Read the model definition and answer for the solid it produces. Units are mm, in the model's axes. Coordinates: 2 decimals unless noted, no trailing zeros. Write each loop counter-clockwise with the first axis right and the second up, starting at its lowest first coordinate (ties: lowest second). Pieces come first, ordered by that corner, then holes. Notation, with made-up numbers: (49, 5.25) -> (84, 5.25) arc R24 cw to (84, 16.25) -> close; hole circle Ø3 at (11, 31.25). An arc over 180 degrees is marked (long way). Return JSON: item names as keys, results as strings.
from build123d import *

# Parameters (mm, degrees)
SKETCH1_R           = 150
BOSS_EXTRUDE1_DEPTH = 10
SKETCH2_R           = 1.73
SKETCH2_R_2         = 2
CUT_EXTRUDE1_DEPTH  = 10


with BuildPart() as part:
    # Sketch1 → Boss-Extrude1 (new body)
    with BuildSketch(Plane(origin=(0, 0, 0), x_dir=(1, 0, 0), z_dir=(0, 1, 0))):
        with Locations(Location((0, 0, 0), (0, 0, 270))):
            Circle(SKETCH1_R)
    extrude(amount=BOSS_EXTRUDE1_DEPTH)

    # Sketch2 → Cut-Extrude1 (cut)
    with BuildSketch(Plane(origin=(0, 10, 0), x_dir=(1, 0, 0), z_dir=(0, 1, 0))):
        with Locations(Location((-14.945, 143.452697854, 0), (0, 0, 270))):
            Circle(SKETCH2_R)
        with Locations(Location((-14.945, 119.392697854, 0), (0, 0, 270))):
            Circle(SKETCH2_R)
        with Locations(Location((14.945, 143.452697854, 0), (0, 0, 90))):
            Circle(SKETCH2_R)
        with Locations(Location((14.945, 119.392697854, 0), (0, 0, 90))):
            Circle(SKETCH2_R)
        with Locations(Location((95.924609368, -72.639098587, 0), (0, 0, 90))):
            Circle(SKETCH2_R)
        with Locations(Location((116.761180583, -84.669098587, 0), (0, 0, 90))):
            Circle(SKETCH2_R)
        with Locations(Location((131.706180583, -58.783599268, 0), (0, 0, 270))):
            Circle(SKETCH2_R)
        with Locations(Location((110.869609368, -46.753599268, 0), (0, 0, 270))):
            Circle(SKETCH2_R)
        with Locations(Location((-110.869609368, -46.753599268, 0), (0, 0, 90))):
            Circle(SKETCH2_R)
        with Locations(Location((-131.706180583, -58.783599268, 0), (0, 0, 90))):
            Circle(SKETCH2_R)
        with Locations(Location((-116.761180583, -84.669098587, 0), (0, 0, 270))):
            Circle(SKETCH2_R)
        with Locations(Location((-95.924609368, -72.639098587, 0), (0, 0, 270))):
            Circle(SKETCH2_R)
        with Locations(Location((-123.062136008, 71.049957351, 0), (0, 0, 270))):
            Circle(SKETCH2_R_2)
        with Locations(Location((123.062136008, 71.049957351, 0), (0, 0, 270))):
            Circle(SKETCH2_R_2)
        with Locations(Location((0, -142.099914702, 0), (0, 0, 270))):
            Circle(SKETCH2_R_2)
    extrude(amount=-CUT_EXTRUDE1_DEPTH, mode=Mode.SUBTRACT)


solid = part.part
1. The part is cut by section C-C (x = 46.5). Determine the outline of the cut face in (y, z).
Taken from the geometry:
{"outline": "(0, -142.61) -> (10, -142.61) -> (10, 142.61) -> (0, 142.61) -> close"}
2. The part is cut by section B-B (z = -40.5). Determine the outline of the cut face in (x, y), then the cut area to 3 significant figures.
Taken from the geometry:
{"outline": "(-144.43, 0) -> (144.43, 0) -> (144.43, 10) -> (-144.43, 10) -> close", "area": "2,890 mm2"}
3. Consider L1, parallel to X at y = 1.5, z = 83.5; L2, parallel to X at y = 2.25, z = 47.5; L3, parallel to Z at x = 116, y = 3.5. Determine where each line is inside the solid, lowest interval first.
Taken from the geometry:
{"L1": "x = -124.61 to -118.04, -115.49 to 115.49, 118.04 to 124.61", "L2": "x = -142.28 to -112.43, -109.31 to 109.31, 112.43 to 142.28", "L3": "z = -95.1 to 83.12, 86.22 to 95.1"}
4. The part is cut by section A-A (y = 1.5). Count the separate pieces of the cut face and the enclosed holes in it, then the cut area to 3 significant figures.
Taken from the geometry:
{"separate pieces": "1", "enclosed holes": "15", "area": "70,500 mm2"}
5. Flat-ended cylindrical pins translate along their axes: pin 1 Ø1.5 at (x, y) = (-60.5, 7) entering from -Z; pin 2 Ø1.5 at (y, z) = (2.5, 114.5) entering from -X; pin 3 Ø6 at (y, z) = (8.5, 68.5) entering from -X; pin 4 Ø4 at (x, z) = (-95.92, 72.64) entering from -Y. Find the tip coordinate at first contact, or state that the pin passes through.
Taken from the geometry:
{"pin 1": "stops at z = -137.59", "pin 2": "stops at x = -97.78", "pin 3": "stops at x = -134.94", "pin 4": "stops at y = 0"}
